Source: three-view drawing plus pictorial views. Frame: mm from the lowest corner of the part. A direction names the side the tool comes from. Coordinates: 2 decimals unless noted, no trailing zeros. Order: outer loops, then holes, each group sorted by start corner. A loop starts at its lowest first (then second) coordinate and runs counter-clockwise, first axis right, second up. Notation, with made-up numbers: (2.5, 39) - (50.5, 39) arc R14 cw to (50.5, 56) - close; hole circle Ø5 at (22, -13.75). An arc over 180 degrees is marked (long way). One line per question, with ' | ' between items.
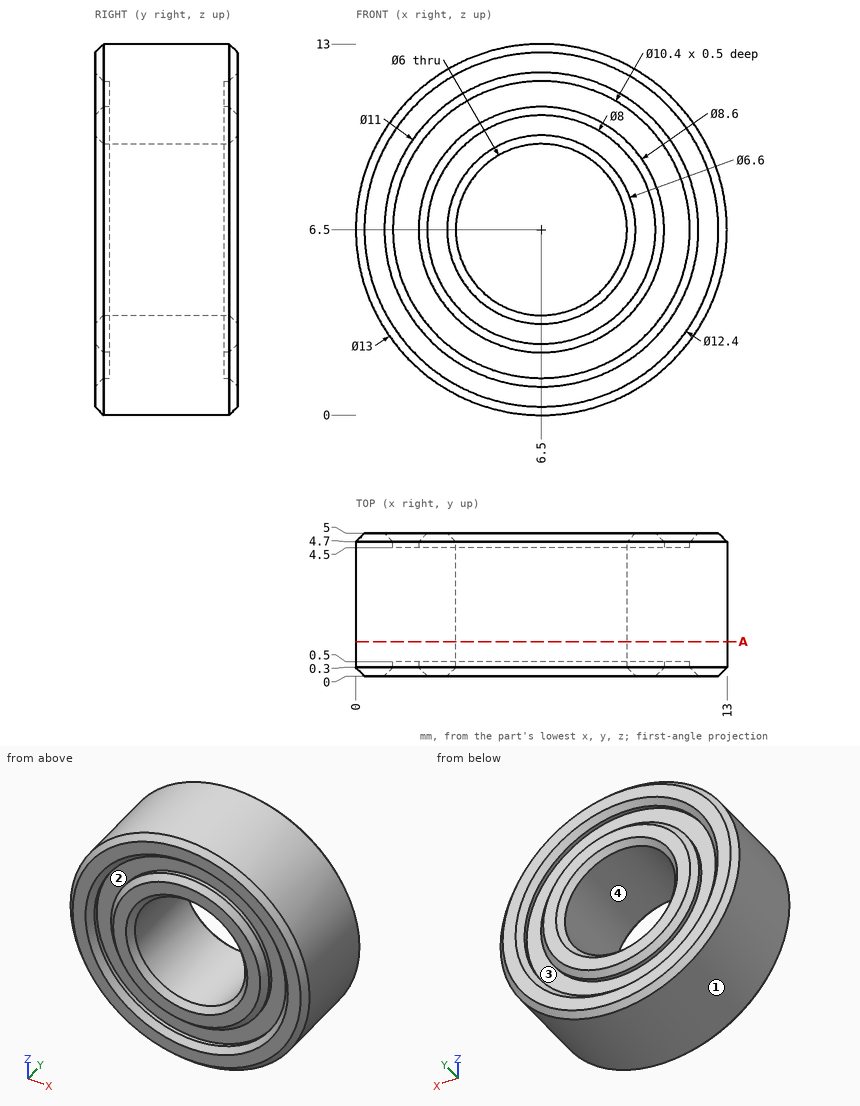
Item 1: Draft query along Z for the marked faces 1 and 2. Return one class per face: released by +Z, released by -Z, zero draft, split by the parting line, or undercut.
Data:
face 1: split by the parting line | face 2: undercut
Item 2: Access query for the marked faces 3 and 4. Directions: +Z, -Z, +X, -X, +Y, -Y. A direction counts if a zero-diameter tool reaches every point of the face in a straight line with its end or side. Return the directions, or none.
Data:
face 3: +Y | face 4: +Y, -Y
Item 3: Ray query, line 1 (Z direction, x = 6.5, y = 4.6); line 2 (Z direction, x = 6.5, y = 0.55); line 3 (Z direction, x = 7.25, y = 1.5). Return the intervals inside material, ascending.
Data:
line 1: 0 to 1.3, 2.2 to 3.5, 9.5 to 10.8, 11.7 to 13 | line 2: 0 to 3.5, 9.5 to 13 | line 3: 0.04 to 3.6, 9.4 to 12.96
Item 4: Section A-A on y = 1.2. Return the cut outline in (x, z), and give its area (3 significant figures).
Data:
outline: circle Ø13 at (6.5, 6.5); hole circle Ø6 at (6.5, 6.5) | area: 104 mm^2
Item 5: Contact query for flat-ended pins moving along their axis: P1, Ø5, axis at x = 6, z = 6, coming from the +Y side; P2, Ø2, axis at x = 8.5, y = 2.5, coming from the -Z side. Output: stop coordinate, or through.
Data:
P1: y = 4.91 | P2: z = 0.08
